from build123d import *

# Parameters (mm, degrees)
F0_R      = 12.7
F1_DEPTH  = 30.1625
F3_W      = 5.6116215229
F3_H      = 22.3266
F3_W_2    = 50.3156215229
F4_DEPTH  = 25.4
F6_DEPTH  = 25.4
F7_R      = 6.35
F8_DEPTH  = 25.4
F9_R      = 7.874
F10_R     = 5.08
F12_DEPTH = 19.05
F13_W     = 19.05
F13_H     = 34.798
F14_DEPTH = 19.05
F15_R     = 5.08
F17_DEPTH = 19.05


with BuildPart() as f1:
    # F0 (on Front) → F1 (new body)
    with BuildSketch(Plane.XZ):
        with BuildLine():
            ThreePointArc((0, -22.352), (15.8052507731, -15.8052507731), (22.352, 0))
            ThreePointArc((22.352, 0), (-15.8052507731, 15.8052507731), (0, -22.352))
        make_face()
        Circle(F0_R, mode=Mode.SUBTRACT)
        with BuildLine():
            Line((194.2084, 0), (22.352, 0))
            ThreePointArc((22.352, 0), (15.8052507731, -15.8052507731), (0, -22.352))
            Line((0, -22.352), (194.2084, -22.352))
            Line((194.2084, -22.352), (194.2084, 0))
        make_face()
    extrude(amount=F1_DEPTH)

    # F2: F1 across plane


with BuildPart() as f1_1:
    add(f1.part)
    add(f1.part.mirror(Plane.XZ))

    # F3 (on face) → F4 (cut)
    with BuildSketch(Plane.XY):
        with Locations((25.1578107615, 0)):
            Rectangle(F3_W, F3_H)
        with Locations((-2.8058107615, 0)):
            Rectangle(F3_W_2, F3_H)
    extrude(amount=-F4_DEPTH, mode=Mode.SUBTRACT)

    # F5 (on face) → F6 (cut)
    with BuildSketch(Plane.XY):
        Polygon((-49.2868088186, -11.1633), (27.9636215229, -11.1633), (27.9636215229, 11.1633), (-41.6799448431, 11.1633), align=None)
    extrude(amount=F6_DEPTH, mode=Mode.SUBTRACT)

    # F7 (on face) → F8 (cut)
    with BuildSketch(Plane.XY):
        with Locations((155.3464, 7.8105)):
            Circle(F7_R)
    extrude(amount=-F8_DEPTH, mode=Mode.SUBTRACT)

    # F9
    f9_edges = [f1_1.edges().sort_by_distance(p)[0] for p in [
        (194.2084, 0, 0),
    ]]
    fillet(f9_edges, radius=F9_R)

    # F10
    f10_edges = [f1_1.edges().sort_by_distance(p)[0] for p in [
        (22.352, -20.6629, 0),
        (22.352, 20.6629, 0),
    ]]
    fillet(f10_edges, radius=F10_R)

    # F11 (on face) → F12 (cut)
    with BuildSketch(Plane.XZ.offset(30.1625)):
        Polygon((117.2464, 0), (85.852, 0), (91.8464, -22.352), (117.2464, -22.352), align=None)
    extrude(amount=-F12_DEPTH, mode=Mode.SUBTRACT)

    # F13 (on face) → F14 (join)
    with BuildSketch(Plane.XZ.offset(30.1625)):
        with Locations((140.5636, 17.399)):
            Rectangle(F13_W, F13_H)
    extrude(amount=-F14_DEPTH)

    # F15
    f15_edges = [f1_1.edges().sort_by_distance(p)[0] for p in [
        (150.0886, -20.6375, 0),
        (150.0886, -20.6375, 34.798),
    ]]
    fillet(f15_edges, radius=F15_R)

    # F16 (on face) → F17 (join)
    with BuildSketch(Plane.XZ.offset(30.1625)):
        with BuildLine():
            ThreePointArc((131.0386, 34.798), (127.4644153616, 16.0823576341), (117.2464, 0))
            Line((117.2464, 0), (131.0386, 0))
            Line((131.0386, 0), (131.0386, 34.798))
        make_face()
    extrude(amount=-F17_DEPTH)


solid = f1_1.part
For this review, take the finished solid that the model builds, in its own axes (mm). A direction names the side the tool comes from. Round coordinates to 2 decimals unless told otherwise and drop trailing zeros. Write each loop counter-clockwise with the first axis right and the second up, starting at its lowest first coordinate (ties: lowest second). Pieces come first, ordered by that corner, then holes. Notation, with made-up numbers: M 84,78 L 109,78 A6 cw 109,84 Z; hole C 72,-6 d11. An arc over 180 degrees is marked long. Write item = value, one per line. Start each with the question number.
(1) The part is to be moulded in two halves that separate along X. For faces 6 (the face through (23.8, -20.5, 1.1)), 7 (the face through (-16.75, 20.53, 14.8)), 8 (the face through (194.208, 0, -15)), say which applies: +X half, -X half, draft (parallel to the pull), parting line (faces both ways), or undercut.
(2) For line 1 along Z through (x, y) = (0, -19.75); line 2 along Y through (x, z) = (-13, -15); line 3 along Z through (x, y) = (-1, -22), list the stretches that pass through material, from the lowest coordinate up.
(3) Clearance check with flat-ended pins moving along their axes: pin 1 Ø6 at (x, z) = (53.5, 2.5) entering from -Y; pin 2 Ø9.5 at (y, z) = (-25, 15.5) entering from +X; pin 3 Ø10 at (x, y) = (155.35, 7.81) entering from -Z; pin 4 Ø6 at (x, y) = (163.5, -6) entering from +Z. State where each tip first meets the part, or that it passes through.
(4) We need section C-C (z = 18). Give the boundary of the cut face in (x, y), then the cut area to 3 significant figures.
(5) We need section A-A (y = -18.5). Give the boundary of the cut face in (x, z).
(6) We need section B-B (x = -9). Give the boundary of the cut face in (y, z).
(7) We need section D-D (y = 25.5). Give the boundary of the cut face in (x, z), then the cut area to 3 significant figures.
(8) For faces 1 (the face through (127.56, -20.77, 16.33)), 2 (the face through (150.089, -21, 17)), 3 (the face through (140, -11.112, 18)), 4 (the face through (101, -11.112, -11)), 5 (the face through (108, 6, 0)), list the 3-axis set-ups (+Z, -Z, +X, -X, +Y, -Y) from which the entire face can be reached by the end or side of a thin tool; tool diameter is ignored.
Results found:
q1.face_6 = undercut
q1.face_7 = parting line
q1.face_8 = +X half
q2.line_1 = -22.35 to -12.7, 12.7 to 22.35
q2.line_2 = -30.16 to -11.16, 11.16 to 30.16
q2.line_3 = -22.33 to -12.66, 12.66 to 22.33
q3.pin_1 = -30.16
q3.pin_2 = 150.09
q3.pin_3 = through
q3.pin_4 = 0
q4.outline = M -13.25,-30.16 L 13.25,-30.16 L 13.25,-11.16 L -13.25,-11.16 Z; M -13.25,11.16 L 13.25,11.16 L 13.25,30.16 L -13.25,30.16 Z; M 128.18,-30.16 L 150.09,-30.16 L 150.09,-11.11 L 128.18,-11.11 Z
q4.area = 1,420 mm²
q5.outline = M 0,-22.35 L 91.85,-22.35 L 85.85,0 L 26.96,0 A5.08 cw 21.97,4.14 A22.35 ccw long Z; M 117.25,-22.35 L 194.21,-22.35 L 194.21,-7.87 A7.87 ccw 186.33,0 L 155.17,0 A5.08 cw 150.09,5.08 L 150.09,29.72 A5.08 ccw 145.01,34.8 L 131.04,34.8 A50.8 cw 117.25,0 Z; hole C 0,0 d25.4
q6.outline = M -30.16,-20.46 L -11.16,-20.46 L -11.16,-8.96 L -30.16,-8.96 Z; M -30.16,8.96 L -11.16,8.96 L -11.16,20.46 L -30.16,20.46 Z; M 11.16,-20.46 L 30.16,-20.46 L 30.16,-8.96 L 11.16,-8.96 Z; M 11.16,8.96 L 30.16,8.96 L 30.16,20.46 L 11.16,20.46 Z
q7.outline = M 0,-22.35 L 194.21,-22.35 L 194.21,-7.87 A7.87 ccw 186.33,0 L 26.96,0 A5.08 cw 21.97,4.14 A22.35 ccw long Z; hole C 0,0 d25.4
q7.area = 5,000 mm²
q8.face_1 = +Z, +Y, -Y
q8.face_2 = +Z, +X, +Y, -Y
q8.face_3 = +Z, +X, -X, +Y
q8.face_4 = +Z, -Y
q8.face_5 = +Z, +Y
